Solid Edge part; units mm, degrees
sketch "Sketch1" plane through (0, 0, 0) normal (0, 0, 1) x (1, 0, 0)
  line L0 (-7.8, -9.1) -> (18.885, -9.1)
  line L1 (45.57, -9.1) -> (18.885, -9.1)
  arc A0 (46.5128, 9.1546) -> (45.57, -9.1) centre (46.57, 0) cw
  line L2 (37.77, 9.1) -> (46.5128, 9.1546)
  line L3 (19.385, 9.1) -> (37.77, 9.1)
  line L4 (19.385, 9.1) -> (18.885, 9.1)
  line L5 (18.385, 9.1) -> (18.885, 9.1)
  line L6 (18.385, 9.1) -> (0, 9.1)
  line L7 (0, 9.1) -> (-8.7428, 9.1546)
  arc A1 (-8.7428, 9.1546) -> (-7.8, -9.1) centre (-8.8, 0) ccw
  line L8 (18.885, 4.1) -> (38.77, 4.1)
  line L9 (38.77, 4.1) -> (40.27, 4.1)
  arc A2 (40.27, 4.1) -> (42.27, 2.1) centre (40.27, 2.1) cw
  line L10 (42.27, 2.1) -> (42.27, -2.1)
  arc A3 (42.27, -2.1) -> (40.27, -4.1) centre (40.27, -2.1) cw
  line L11 (40.27, -4.1) -> (18.885, -4.1)
  line L12 (-2.5, -4.1) -> (18.885, -4.1)
  arc A4 (-4.5, -2.1) -> (-2.5, -4.1) centre (-2.5, -2.1) ccw
  line L13 (-4.5, 2.1) -> (-4.5, -2.1)
  arc A5 (-2.5, 4.1) -> (-4.5, 2.1) centre (-2.5, 2.1) ccw
  line L14 (-1, 4.1) -> (-2.5, 4.1)
  line L15 (18.885, 4.1) -> (-1, 4.1)
extrude "Protrusion1" add sketch "Sketch1" along normal blind 16
sketch "Sketch2" plane through (-4.5, 0, 8) normal (1, 0, 0) x (0, 1, 0)
  line L0 (0, 6.6171) -> (3.7944, 2.6879)
  arc A0 (3.7944, 2.6879) -> (4.225, 1.9421) centre (0, 0) cw
  line L1 (4.225, 1.9421) -> (4.225, 0)
  line L2 (4.225, -1.9421) -> (4.225, 0)
  arc A1 (4.225, -1.9421) -> (3.7944, -2.6879) centre (0, 0) cw
  line L3 (3.7944, -2.6879) -> (2.1125, -3.659)
  line L4 (0.4306, -4.63) -> (2.1125, -3.659)
  arc A2 (0.4306, -4.63) -> (-0.4306, -4.63) centre (0, 0) cw
  line L5 (-0.4306, -4.63) -> (-2.1125, -3.659)
  line L6 (-3.7944, -2.6879) -> (-2.1125, -3.659)
  arc A3 (-3.7944, -2.6879) -> (-4.225, -1.9421) centre (0, 0) cw
  line L7 (-4.225, -1.9421) -> (-4.225, 0)
  line L8 (-4.225, 1.9421) -> (-4.225, 0)
  arc A4 (-4.225, 1.9421) -> (-3.7944, 2.6879) centre (0, 0) cw
  line L9 (-3.7944, 2.6879) -> (0, 6.6171)
extrude "ExtrudedCutout_1" cut sketch "Sketch2" against normal blind 3.3 and the other way blind 5
sketch "Sketch3" plane through (-4.5, 0, 8) normal (1, 0, 0) x (0, 1, 0)
  line L0 (0, 3.8868) -> (-1.9422, 1.8756)
  line L1 (1.9422, 1.8756) -> (0, 3.8868)
  arc A0 (1.9422, 1.8756) -> (-1.9422, 1.8756) centre (0, 0) cw
extrude "Cutout1" cut sketch "Sketch3" against normal through all
sketch "Sketch4" plane through (18.385, 9.1, 8) normal (0, 1, 0) x (-1, 0, 0)
  arc A0 (-13.5272, 1.8756) -> (-9.6428, 1.8756) centre (-11.585, 0) ccw
  line L0 (-11.585, 3.8868) -> (-9.6428, 1.8756)
  line L1 (-13.5272, 1.8756) -> (-11.585, 3.8868)
extrude "Cutout2" cut sketch "Sketch4" against normal through all
mirror "Mirror1" about plane through (18.885, 0, 0) normal (1, 0, 0) of "ExtrudedCutout_1", "Cutout1", "Cutout2"
properties material "ABS Plastic, medium impact"
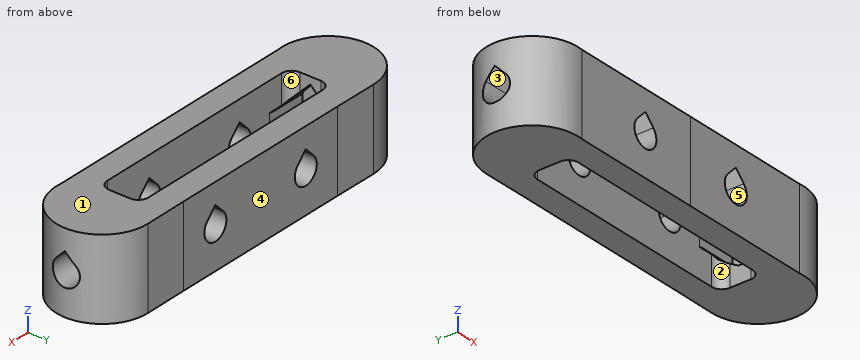
Input: part model. Units: mm. Frame: model coordinates. Face numbers are marked on the shaded views. A direction names the side the tool comes from. Give positions to 0.01 mm unless a question says otherwise; leave off trailing zeros. Write each loop counter-clockwise with the first axis right and the second up, starting at its lowest first coordinate (ties: lowest second). Pieces come first, ordered by that corner, then holes. Notation, with made-up numbers: (0, 77) - (7, 77) arc R35 cw to (7, 114) - close; hole circle Ø7 at (-27.5, 75). An arc over 180 degrees is marked (long way). Write item = value, one per line. Start each with the question number.
1. Mould query, pull axis Y, two halves, no side actions, for the marked faces 4, 5 and 6. Classes: released by +Y, released by -Y, zero draft, split by the parting line, or undercut.
2. Ray query, L1, parallel to X at y = -0.5, z = 14; L2, parallel to X at y = -6.9, z = 8; L3, parallel to X at y = -8, z = 6. Return the intervals inside material, ascending.
3. Section query A-A, the plane z = 2. Output: boundary loops of the cut face in (x, y) (3 decimals), then the cut area to 3 significant figures.
4. Section query B-B, the plane y = -7.5. Output: boundary loops of the cut face in (x, z), then the cut area to 3 significant figures.
5. Access query for the marked faces 1, 2 and 3. Directions: +Z, -Z, +X, -X, +Y, -Y. A direction counts if a zero-diameter tool reaches every point of the face in a straight line with its end or side. Return the directions, or none.
6. First-contact query: pin 1 Ø8 at (x, z) = (37.5, 7.5) entering from -Y; pin 2 Ø2 at (x, z) = (9.5, 9) entering from +Y; pin 3 Ø2.5 at (y, z) = (-1, 9.5) entering from -X. Flat tips, straight axial feed; report the tip coordinate or a pass-through.
7. Section query C-C, the plane y = 1.25. Output: boundary loops of the cut face in (x, z), then the cut area to 3 significant figures.
Check sheet entries:
q1.face_4 = released by +Y
q1.face_5 = zero draft
q1.face_6 = undercut
q2.L1 = -17.94 to -7.8, 45.57 to 55.71
q2.L2 = -14.82 to 5.1, 10.5 to 27.27, 32.67 to 52.59
q2.L3 = -13.25 to 5.99, 9.61 to 28.16, 31.78 to 51.02
q3.outline = (-8.743, 9.155) arc R9.155 ccw (long way) to (-7.8, -9.1) - (45.57, -9.1) arc R9.155 ccw (long way) to (46.513, 9.155) - (37.77, 9.1) - (0, 9.1) - close; hole (-4.5, -2.1) arc R2 ccw to (-2.5, -4.1) - (40.27, -4.1) arc R2 ccw to (42.27, -2.1) - (42.27, 2.1) arc R2 ccw to (40.27, 4.1) - (-2.5, 4.1) arc R2 ccw to (-4.5, 2.1) - close
q3.area = 892 mm2
q4.outline = (-14.05, 0) - (51.82, 0) - (51.82, 16) - (-14.05, 16) - close; hole (5.86, 9.88) arc R2.7 ccw (long way) to (9.74, 9.88) - (7.8, 11.89) - close; hole (28.03, 9.88) arc R2.7 ccw (long way) to (31.91, 9.88) - (29.97, 11.89) - close
q4.area = 1,000 mm2
q5.face_1 = +Z, +X, -X, +Y, -Y
q5.face_2 = +Z, -Z
q5.face_3 = +X, -X
q6.pin_1 = -9.1
q6.pin_2 = 9.1
q6.pin_3 = -17.89
q7.outline = (-17.87, 0) - (-4.5, 0) - (-4.5, 3.84) - (-7.8, 3.84) - (-7.8, 5.61) - (-17.87, 5.61) - close; (-17.87, 10.59) - (-7.8, 10.59) - (-7.8, 13.32) - (-4.5, 13.32) - (-4.5, 16) - (-17.87, 16) - close; (42.27, 0) - (55.64, 0) - (55.64, 5.61) - (45.57, 5.61) - (45.57, 3.84) - (42.27, 3.84) - close; (42.27, 13.32) - (45.57, 13.32) - (45.57, 10.59) - (55.64, 10.59) - (55.64, 16) - (42.27, 16) - close
q7.area = 265 mm2
